Answer from the drawing. Dimensions are ordinates in mm from the lowest x, y and z of the part. A direction names the side the tool comes from. Coordinates: 2 decimals unless noted, no trailing zeros. Write each loop counter-clockwise with the first axis right and the second up, starting at its lowest first coordinate (ties: lowest second). Pieces come first, ordered by that corner, then holes. Notation, with made-up numbers: (88.25, 51) - (141.25, 51) arc R24 cw to (141.25, 70) - close; hole circle Ø9 at (-19.75, 65). An arc over 180 degrees is marked (long way). Use a Markdown table: item, result.
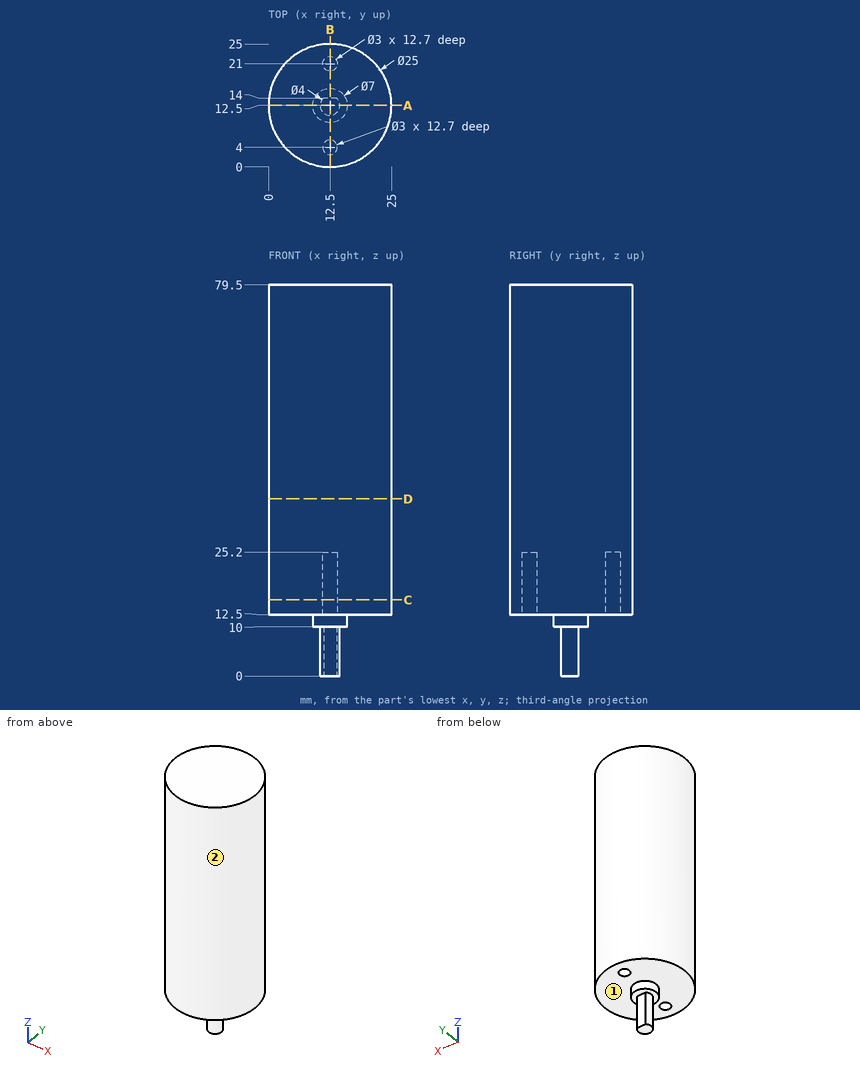
(1) For the marked faces 1 and 2, determine the directions among +Z, -Z, +X, -X, +Y, -Y from which every point of the face is accessible in a straight line to the end or side of a thin tool.
Report:
| item | result |
|---|---|
| face 1 | -Z |
| face 2 | +Z, -Z |
(2) A cutting plane is placed at D-D, the plane z = 36. Write down the section's boundary in (x, y).
Report:
| item | result |
|---|---|
| outline | circle Ø25 at (12.5, 12.5) |
(3) A cutting plane is placed at B-B, the plane x = 12.5. Write down the section's boundary in (y, z), and give its area (3 significant figures).
Report:
| item | result |
|---|---|
| outline | (0, 12.5) - (2.5, 12.5) - (2.5, 25.2) - (5.5, 25.2) - (5.5, 12.5) - (9, 12.5) - (9, 10) - (10.5, 10) - (10.5, 0) - (14, 0) - (14, 10) - (16, 10) - (16, 12.5) - (19.5, 12.5) - (19.5, 25.2) - (22.5, 25.2) - (22.5, 12.5) - (25, 12.5) - (25, 79.5) - (0, 79.5) - close |
| area | 1,650 mm² |
(4) A cutting plane is placed at C-C, the plane z = 15.5. Write down the section's boundary in (x, y), and give its area (3 significant figures).
Report:
| item | result |
|---|---|
| outline | circle Ø25 at (12.5, 12.5); hole circle Ø3 at (12.5, 4); hole circle Ø3 at (12.5, 21) |
| area | 477 mm² |
(5) A cutting plane is placed at A-A, the plane y = 12.5. Write down the section's boundary in (x, z).
Report:
| item | result |
|---|---|
| outline | (0, 12.5) - (9, 12.5) - (9, 10) - (10.5, 10) - (10.5, 0) - (14.5, 0) - (14.5, 10) - (16, 10) - (16, 12.5) - (25, 12.5) - (25, 79.5) - (0, 79.5) - close |
(6) Each of these flat-tipped pins is pushed along its axis until it touches: P1, Ø8, axis at y = 4.5, z = 18, coming from the -X side; P2, Ø2, axis at x = 6, z = 13, coming from the -Y side (3 decimals); P3, Ø8, axis at y = 3, z = 23.5, coming from the -X side (3 decimals). Where does it stop, or does it pass through?
Report:
| item | result |
|---|---|
| P1 | stops at x = 0.66 |
| P2 | stops at y = 1.275 |
| P3 | stops at x = 1.275 |
(7) Straight lines are drawn through the part: L1, parallel to Y at x = 12.5, z = 21; L2, parallel to Z at x = 20.25, y = 6; L3, parallel to X at y = 5, z = 73. For each, find the intervals that lie inside material, in ascending order.
Report:
| item | result |
|---|---|
| L1 | y = 0 to 2.5, 5.5 to 19.5, 22.5 to 25 |
| L2 | z = 12.5 to 79.5 |
| L3 | x = 2.5 to 22.5 |
